Autodesk Inventor part; units mm, degrees
ref_plane "YZ Plane" through (0, 0, 0) normal (1, 0, 0) x (0, 1, 0)
ref_plane "XZ Plane" through (0, 0, 0) normal (0, 1, 0) x (-1, 0, 0)
ref_plane "XY Plane" through (0, 0, 0) normal (0, 0, 1) x (1, 0, 0)
sketch "Sketch1" plane through (0, 0, 0) normal (0, 1, 0) x (-1, 0, 0)
  circle A0 centre (0, 0) radius 60
  circle A1 centre (60, 0) radius 4
  circle A2 centre (-30, 51.9615) radius 4
  circle A3 centre (-30, -51.9615) radius 4
  circle A4 centre (-30, 51.9615) radius 15
  circle A5 centre (-30, -51.9615) radius 15
  circle A6 centre (60, 0) radius 15
  line L0 (21, -21) -> (-21, -21)
  line L1 (-21, -21) -> (-21, 21)
  line L2 (-21, 21) -> (21, 21)
  line L3 (21, 21) -> (21, -21)
  line L4 (21, -21) -> (-21, 21) construction
  line L5 (-21, -21) -> (21, 21) construction
  circle A7 centre (0, 0) radius 5
  line L6 (60, 15) -> (25.632, 15)
  line L7 (60, -15) -> (25.632, -15)
  circle A8 centre (0, 0) radius 29.6985
  circle A9 centre (28.3546, 20) radius 5
  circle A10 centre (28.3546, -20) radius 5
  circle A11 centre (-31.4978, 14.5558) radius 5
  line L8 (-42.9904, 44.4615) -> (-25.8064, 14.698)
  line L9 (-17.0096, 59.4615) -> (0.1744, 29.698)
  circle A12 centre (3.1432, 34.5558) radius 5
  circle A13 centre (3.1432, -34.5558) radius 5
  line L10 (-17.0096, -59.4615) -> (0.1744, -29.698)
  line L11 (-42.9904, -44.4615) -> (-25.8064, -14.698)
  circle A14 centre (-31.4978, -14.5558) radius 5
  point P0 (16, -16)
  point P1 (16, 16)
  point P2 (-16, 16)
  point P3 (-16, -16)
  point P4 (-16.174, 57.7789)
  point P5 (-41.951, 42.8966)
  point P6 (-42.0378, 42.8115)
  point P7 (-25.8064, 14.698)
  point P8 (-25.8064, -14.698)
  point P9 (-42.0378, -42.8115)
  point P10 (-41.951, -42.8966)
  point P11 (-16.174, -57.7789)
  point P12 (-16.057, -57.8115)
  point P13 (58.0948, -15)
  point P14 (58.125, -14.8824)
  point P15 (58.125, 14.8824)
  point P16 (58.0948, 15)
  point P17 (-16.057, 57.8115)
  point P18 (-26.4712, -53.8449)
  point P19 (-33.3955, -49.8472)
  dimension "d0" = 120
  dimension "d2" = 8
  dimension "d5" = 360
  dimension "d7" = 30
  dimension "d8" = 30
  dimension "d9" = 30
  dimension "d10" = 42
  dimension "d11" = 42
  dimension "d12" = 10
  dimension "d13" = 32
  dimension "d14" = 16
  dimension "d15" = 16
  dimension "d16" = 32
  dimension "d17" = 10
  dimension "d18" = 10
  dimension "d21" = 360
extrude "Extrusion1" add sketch "Sketch1" along normal blind 5 contours A1 A0 A6 | A0 A6 A1 | A6 A0 L7 A8 L6 | A0 L6 A6 | A6 L7 A0 | L9 A8 L8 A0 A4 | A0 A4 L9 | L10 A5 A0 | A0 A5 L11 A8 L10 | A4 A0 A2 | A0 A2 A4 | A8 L3 | A5 A0 A3 | A0 A3 A5 | A4 A0 L8 | A8 L2 | L3 L0 L1 L2 | L11 A0 A5 | A8 L0 | L1 A8
sketch "Sketch3" plane through (0, 5, 0) normal (0, 1, 0) x (1, 0, 0)
  point P0 (0, 0)
  point P1 (0, 18.5)
  point P2 (0, -18.5)
  dimension "d36" = 37
  dimension "d37" = 18.5
hole "Hole2" at (0, 5, -18.5) at (0, 5, 18.5) direction (0, -1, 0) diameter 5 end through all
sketch "Sketch4" plane through (0, 5, 0) normal (0, 1, 0) x (1, 0, 0)
  circle A0 centre (30, 51.9615) radius 4
  circle A1 centre (-60, 0) radius 4
  circle A2 centre (30, -51.9615) radius 4
  point P0 (0, 0)
  point P1 (-60, -9)
  point P2 (-60, 9)
  point P3 (26.4712, 53.8449)
  point P4 (33.3955, 49.8472)
  dimension "d45" = 18
  dimension "d46" = 9
hole "Hole3" at (-60, 5, 9) at (-60, 5, -9) direction (0, -1, 0) diameter 4 end through all
pattern_circular "Circular Pattern1" count 3 over 360 about axis through (0, 0, 0) along (0, 1, 0) of "Hole3"
properties part number "De_Tren_Cung" material "Aluminum 6061"
Can you work these out from the model? Positions are in its coordinate system, mm. A direction names the side the tool comes from. Coordinates: 2 decimals unless noted, no trailing zeros. Order: outer loops, then holes, each group sorted by start corner. A loop starts at its lowest first (then second) coordinate and runs counter-clockwise, first axis right, second up.
1. I need wall thicknesses on line 1 (Z direction, x = -58.5, y = 0.8); line 2 (X direction, y = 0.85, z = 2); line 3 (Z direction, x = 0, y = 2.75). Which ranges of each line are inside material? Lowest first, please.
2. For faces 4 (the face through (1.08, 2.46, 4.88)), 5 (the face through (-43, 2, -15)), which set-ups out of +Z, -Z, +X, -X, +Y, -Y let a thin tool reach every point of the face, with its end or its side?
3. If we section it at A-A (z = 0): Please give me the cut outline in (x, y).
4. I'm going to push flat-ended pins straight in: pin 1 (1 mm diameter, centred on x = -14, y = 3, fed in from -Z); pin 2 (1.5 mm diameter, centred on x = -62, y = 4, fed in from +Z); pin 3 (1.5 mm diameter, centred on x = -37.5, y = 3.5, fed in from +Z). Where does each tip first touch, or does it pass through?
5. Thinking about a two-plate mould opening in Z: for faces 1 (the face through (36.443, 2.465, -48.936)), 2 (the face through (-75, 2, 0)), 3 (the face through (13, 5, 1)), which applies, +Z half, -Z half, draft (parallel to the pull), parting line (faces both ways), or undercut?
6. If we section it at D-D (x = -15.5): Please give me the cut outline in (y, z), then the cut area to 3 significant figures.
7. If we section it at C-C (z = -18.5): Please give me the cut outline in (x, y).
Entries:
1. line 1: z = -15 to -10.32, -7.68 to -3.71, 3.71 to 7.68, 10.32 to 15
1. line 2: x = -74.87 to -63.46, -56.54 to -4.58, 4.58 to 29.63
1. line 3: z = -30 to -21, -16 to -5, 5 to 16, 21 to 30
2. face 4: +Y, -Y
2. face 5: -Z, -X, +Y, -Y
3. outline: (-75, 0) - (-64, 0) - (-64, 5) - (-75, 5) - close; (-56, 0) - (-5, 0) - (-5, 5) - (-56, 5) - close; (5, 0) - (29.7, 0) - (29.7, 5) - (5, 5) - close
4. pin 1: stops at z = -26.45
4. pin 2: stops at z = 14.95
4. pin 3: stops at z = 15
5. face 1: undercut
5. face 2: parting line
5. face 3: draft
6. outline: (0, -25.33) - (5, -25.33) - (5, 25.33) - (0, 25.33) - close
6. area: 253 mm2
7. outline: (-23.23, 0) - (-2.5, 0) - (-2.5, 5) - (-23.23, 5) - close; (2.5, 0) - (28, 0) - (28, 5) - (2.5, 5) - close
